Autodesk Inventor part; units mm, degrees
ref_plane "YZ Plane" through (0, 0, 0) normal (1, 0, 0) x (0, 1, 0)
ref_plane "XZ Plane" through (0, 0, 0) normal (0, 1, 0) x (-1, 0, 0)
ref_plane "XY Plane" through (0, 0, 0) normal (0, 0, 1) x (1, 0, 0)
sketch "Skizze1" plane through (0, 0, 0) normal (0, 1, 0) x (-1, 0, 0)
  line L0 (-50, 40) -> (50, 40)
  line L1 (50, 40) -> (50, -40)
  line L2 (50, -40) -> (-50, -40)
  line L3 (-50, -40) -> (-50, 40)
  line L4 (-50, 40) -> (50, -40) construction
  line L5 (50, 40) -> (-50, -40) construction
  point P0 (0, 0)
  dimension "d0" = 100
  dimension "d1" = 80
extrude "Extrusion1" add sketch "Skizze1" along normal blind 5
sketch "Skizze2" plane through (0, 5, 0) normal (0, 1, 0) x (1, 0, 0)
  line L0 (-50, -40) -> (50, -40)
  line L1 (50, -40) -> (50, 40)
  line L2 (50, 40) -> (-50, 40)
  line L3 (-50, 40) -> (-50, -40)
  line L4 (-45, -35) -> (45, -35)
  line L5 (45, -35) -> (45, 35)
  line L6 (45, 35) -> (-45, 35)
  line L7 (-45, 35) -> (-45, -35)
  line L8 (-45, -35) -> (45, 35) construction
  line L9 (45, -35) -> (-45, 35) construction
  point P0 (0, 0)
  dimension "d4" = 90
  dimension "d5" = 70
extrude "Extrusion2" add sketch "Skizze2" along normal blind 15
properties part number "top"
The model under review builds one solid part; all positions refer to its coordinate system, in mm. A direction names the side the tool comes from. Coordinates: 2 decimals unless noted, no trailing zeros. Write each loop counter-clockwise with the first axis right and the second up, starting at its lowest first coordinate (ties: lowest second). Pieces come first, ordered by that corner, then holes.
1) To check wall thickness, follow probe 1 along Z at (x, y) = (-38, 17.75); probe 2 along X at (y, z) = (8.5, -22.5); probe 3 along Y at (x, z) = (15.5, -22.5). State the ranges of each line that lie inside material, in increasing order.
2) The part is to be moulded in two halves that separate along X. For faces 3 (the face through (-50, 10, 1)), 4 (the face through (1, 12, -35)), 5 (the face through (50, 10, -1)), say which applies: pulls with the +X half, pulls with the -X half, needs draft (parallel to the pull), parting line crosses it, or undercut.
3) Machinability: for faces 1 (the face through (1, 0, 1)), 2 (the face through (45, 12, 0)), which of the approach directions +Z, -Z, +X, -X, +Y, -Y give a long, thin tool a straight path to every point of the face, cutting with its end or side? Answer none if there is none.
4) We need section A-A on y = 15.25. State the section outline as (x, z) points, then the cut area to 3 significant figures.
5) We need section C-C on x = -7. State the section outline as (y, z) points, then the cut area to 3 significant figures.
6) We need section B-B on z = -16. State the section outline as (x, y) points, then the cut area to 3 significant figures.
7) Clearance check with flat-ended pins moving along their axes: pin 1 Ø6 at (x, z) = (-39.5, -9.5) entering from +Y; pin 2 Ø4 at (x, z) = (2, 18) entering from -Y. State where each tip first meets the part, or that it passes through.
Answer list:
1. probe 1: z = -40 to -35, 35 to 40
1. probe 2: x = -50 to -45, 45 to 50
1. probe 3: y = 0 to 5
2. face 3: pulls with the -X half
2. face 4: undercut
2. face 5: pulls with the +X half
3. face 1: +Z, -Z, +X, -X, -Y
3. face 2: +Y
4. outline: (-50, -40) - (50, -40) - (50, 40) - (-50, 40) - close; hole (-45, -35) - (45, -35) - (45, 35) - (-45, 35) - close
4. area: 1,700 mm2
5. outline: (0, -40) - (20, -40) - (20, -35) - (5, -35) - (5, 35) - (20, 35) - (20, 40) - (0, 40) - close
5. area: 550 mm2
6. outline: (-50, 0) - (50, 0) - (50, 20) - (45, 20) - (45, 5) - (-45, 5) - (-45, 20) - (-50, 20) - close
6. area: 650 mm2
7. pin 1: stops at y = 5
7. pin 2: stops at y = 0
